Autodesk Inventor part; units mm, degrees
ref_plane "YZ Plane" through (0, 0, 0) normal (1, 0, 0) x (0, 1, 0)
ref_plane "XZ Plane" through (0, 0, 0) normal (0, 1, 0) x (-1, 0, 0)
ref_plane "XY Plane" through (0, 0, 0) normal (0, 0, 1) x (1, 0, 0)
sketch "Sketch4" plane through (0, 0, 0) normal (0, 1, 0) x (-1, 0, 0)
  circle A0 centre (0, 0) radius 5
extrude "Extrusion2" add sketch "Sketch4" along normal mid plane 10
fillet "Fillet5" radius 4 1 edges at (5, 5, 0)
sketch "Sketch14" plane through (0, -5, 0) normal (0, -1, 0) x (1, 0, 0)
  circle A0 centre (0, 0) radius 1
hole "Hole6" at (0, -5, 0) direction (0, 1, 0) diameter 3 depth 7
sketch "Sketch15" plane through (0, 0, 0) normal (1, 0, 0) x (0, 1, 0)
  line L0 (-5, 5) -> (-5, -5)
  point P0 (0, 0)
  point P1 (-1.5, 0)
  dimension "d109" = 3.5
hole "Hole7" at (0, -1.5, 0) direction (-1, 0, 0) diameter 2.85 depth 10.4
properties part number "Top Lock Cap" material "Mild Steel S355 J2"
Design review of the part built by this model. Coordinates are the model's own, in mm. A direction names the side the tool comes from. Coordinates: 2 decimals unless noted, no trailing zeros. Loops run counter-clockwise (first coordinate to the right, second up) from the corner with the lowest first, then second, coordinate; pieces in that order, holes last. Notation, with made-up numbers: M 9,-9.5 L 68,-9.5 A33 cw 68,22.5 Z; hole C 79.5,84 d2. An arc over 180 degrees is marked long. Answer as CSV lines item,"result".
Item 1: Add section A-A on y = -3.5. State the section outline as (x, z) points, plus the area to 3 significant figures.
Answer list:
outline,"C 0,0 d10; hole C 0,0 d3"
area,"71.5 mm²"
Item 2: For probe 1 along Z at (x, y) = (0, -3.25); probe 2 along Y at (x, z) = (0, 0.5); probe 3 along Z at (x, y) = (-3.95, -1.5) (3 decimals), list the stretches that pass through material, from the lowest coordinate up.
Answer list:
probe 1,"-5 to -1.5, 1.5 to 5"
probe 2,"2 to 5"
probe 3,"-3.066 to -1.425, 1.425 to 3.066"
Item 3: For P1, Ø1.5, axis at x = -2.5, y = -2.5, coming from the -Z side; P2, Ø4, axis at x = -3, z = -2, coming from the +Y side; P3, Ø1.5, axis at x = 3, z = 1.5, coming from the +Y side; P4, Ø6, axis at x = 1.5, y = -2, coming from the +Z side, all flat-tipped, find the tip position at first contact; note any pin that passes through.
Answer list:
P1,"z = -4.68"
P2,"y = 4.95"
P3,"y = 4.66"
P4,"z = 5"
Item 4: The part is to be moulded in two halves that separate along Z. For faces 4 (the face through (1.08, -2.04, 4.88)), 5 (the face through (1.464, -1.451, 0.325)), 6 (the face through (1.2, -5, 1.2)), say which applies: pulls with the +Z half, pulls with the -Z half, needs draft (parallel to the pull), parting line crosses it, or undercut.
Answer list:
face 4,"parting line crosses it"
face 5,"undercut"
face 6,"needs draft"
Item 5: Machinability: for faces 1 (the face through (-3.27, -1.93, -1.36)), 2 (the face through (0, 5, 0)), 3 (the face through (0, 2, 0)), which of the approach directions +Z, -Z, +X, -X, +Y, -Y give a long, thin tool a straight path to every point of the face, cutting with its end or side? Answer none if there is none.
Answer list:
face 1,"-X"
face 2,"+Z, -Z, +X, -X, +Y"
face 3,"-Y"
